Can you work these out from the model? Positions are in its coordinate system, mm. A direction names the side the tool comes from. Round coordinates to 2 decimals unless told otherwise and drop trailing zeros. Loops run counter-clockwise (first coordinate to the right, second up) from the corner with the lowest first, then second, coordinate; pieces in that order, holes last.
```python
from build123d import *

# Parameters (mm, degrees)
SKETCH_W              = 115
SKETCH_H              = 25
PAD_DEPTH             = 3
PAD001_DEPTH          = 3
SKETCH002_W           = 115
SKETCH002_H           = 25
SKETCH002_W_2         = 96
SKETCH002_H_2         = 3
PAD002_DEPTH          = 3
SKETCH003_R           = 0.825
POCKET_DEPTH          = 245.060315
POLARPATTERN_COUNT    = 2
POLARPATTERN001_COUNT = 2
POLARPATTERN002_COUNT = 2
FILLET_R              = 2
SKETCH004_R           = 12.75
POCKET001_DEPTH       = 3
POCKET002_DEPTH       = 3
FILLET001_R           = 0.4
FILLET002_R           = 2


with BuildPart() as part:
    # Sketch → Pad (new body)
    with BuildSketch(Plane.XY):
        Rectangle(SKETCH_W, SKETCH_H)
    extrude(amount=PAD_DEPTH)

    # Sketch001 (on Face6 of Pad) → Pad001 (join)
    with BuildSketch(Plane.XY.offset(3)):
        Polygon((-57.5, 12.5), (57.5, 12.5), (57.5, 4), (50, 4), (50, 5), (-50, 5), (-50, 4), (-57.5, 4), align=None)
        Polygon((-57.5, -12.5), (57.5, -12.5), (57.5, -4), (50, -4), (50, -5), (-50, -5), (-50, -4), (-57.5, -4), align=None)
    extrude(amount=PAD001_DEPTH)

    # Sketch002 (on Face12 of Pad001) → Pad002 (join)
    with BuildSketch(Plane.XY.offset(6)):
        Rectangle(SKETCH002_W, SKETCH002_H)
        Rectangle(SKETCH002_W_2, SKETCH002_H_2, mode=Mode.SUBTRACT)
    extrude(amount=PAD002_DEPTH)

    # Sketch003 (on Face26 of Pad002) → Pocket (cut, through all)
    with BuildSketch(Plane.XY.offset(9)):
        with Locations((-52.5, 7.5)):
            Circle(SKETCH003_R)
    pocket = extrude(amount=-POCKET_DEPTH, mode=Mode.SUBTRACT)

    # PolarPattern: Pocket ×2 about axis
    polarpattern_axis = Axis((0, 0, 0), (0, 1, 0))
    for i in range(1, POLARPATTERN_COUNT):
        add(pocket.rotate(polarpattern_axis, i * 360 / POLARPATTERN_COUNT), mode=Mode.SUBTRACT)

    # PolarPattern001: Pocket ×2 about axis
    polarpattern001_axis = Axis((0, 0, 0), (1, 0, 0))
    for i in range(1, POLARPATTERN001_COUNT):
        add(pocket.rotate(polarpattern001_axis, i * 360 / POLARPATTERN001_COUNT), mode=Mode.SUBTRACT)

    # PolarPattern002: Pocket ×2 about axis
    polarpattern002_axis = Axis((0, 0, 9), (0, 0, 1))
    for i in range(1, POLARPATTERN002_COUNT):
        add(pocket.rotate(polarpattern002_axis, i * 360 / POLARPATTERN002_COUNT), mode=Mode.SUBTRACT)

    # Fillet
    fillet_edges = [part.edges().sort_by_distance(p)[0] for p in [
        (57.5, 12.5, 7.5),
        (57.5, 12.5, 4.5),
        (57.5, 12.5, 1.5),
        (57.5, -12.5, 7.5),
        (-57.5, 12.5, 7.5),
        (-57.5, -12.5, 7.5),
    ]]
    fillet(fillet_edges, radius=FILLET_R)

    # Sketch004 (on Face2 of Fillet) → Pocket001 (cut)
    with BuildSketch(Plane(origin=(0, 0, 0), x_dir=(1, 0, 0), z_dir=(0, 0, -1))):
        with Locations((0, -4.31247)):
            Circle(SKETCH004_R)
    extrude(amount=-POCKET001_DEPTH, mode=Mode.SUBTRACT)

    # Sketch005 (on Face2 of Pocket001) → Pocket002 (cut)
    with BuildSketch(Plane(origin=(0, 0, 0), x_dir=(1, 0, 0), z_dir=(0, 0, -1))):
        Polygon((0.086598, 10.584693), (-49.736099, 10.584693), (-49.736099, 6.30074), (-54.94091, 3.161258), (-54.94091, -2.621142), (-51.300568, -2.835279), (-51.086433, 1.161956), (-44.025761, 5.729707), (0.086598, 5.729707), align=None)
    extrude(amount=-POCKET002_DEPTH, mode=Mode.SUBTRACT)

    # Fillet001
    fillet001_edges = [part.edges().sort_by_distance(p)[0] for p in [
        (-7.856028, -5.729707, 1.5),
    ]]
    fillet(fillet001_edges, radius=FILLET001_R)

    # Fillet002
    fillet002_edges = [part.edges().sort_by_distance(p)[0] for p in [
        (0.086598, -8.437236, 1.5),
    ]]
    fillet(fillet002_edges, radius=FILLET002_R)


solid = part.part
```
(1) Suppose I cut it at A-A (z = 4.25). Write out the boundary of the cut face in (x, y) (3 decimals), then the cut area to 3 significant figures.
(2) For pin 1 (5 mm diameter, centred on x = 2.5, y = 0, fed in from -Z); pin 2 (8.5 mm diameter, centred on x = -4.5, y = 7, fed in from -Z), each with a flat end and sliding along its axis, tell me the tip position at first contact or that it passes through.
(3) Suppose I cut it at B-B (x = -4.5). Write out the boundary of the cut face in (y, z), then the cut area to 3 significant figures.
(4) Which directions (+Z, -Z, +X, -X, +Y, -Y) give clear straight access to the entire face, cutting with the end or side of a thin tool? Please do faces 5 (the flat face through (54, -4, 4)), 6 (the flat face through (-24, -10.585, 1)), 7 (the flat face through (33, 0, 3)).
(5) We'd pull the mould along Z, two halves only. Please class faces 1 (the flat face through (-1, -1.5, 7)), 2 (the flat face through (-1, 3, 9)), 3 (the flat face through (-1, 2, 6)), 4 (the flat face through (1, 5, 4)): released by +Z, released by -Z, zero draft, split by the parting line, or undercut.
(6) If I drill on line 1 (X direction, y = -7.5, z = 5) (3 decimals); line 2 (Y direction, x = 52.5, z = 6.75) (3 decimals); line 3 (Y direction, x = -52.5, z = 4) (3 decimals), over which ranges is the centre line in solid material (lowest first)?
Check result:
1. outline: (-57.5, -10.5) arc R2 ccw to (-55.5, -12.5) - (55.5, -12.5) arc R2 ccw to (57.5, -10.5) - (57.5, -4) - (50, -4) - (50, -5) - (-50, -5) - (-50, -4) - (-57.5, -4) - close; (-57.5, 4) - (-50, 4) - (-50, 5) - (50, 5) - (50, 4) - (57.5, 4) - (57.5, 10.5) arc R2 ccw to (55.5, 12.5) - (-55.5, 12.5) arc R2 ccw to (-57.5, 10.5) - close; hole circle Ø1.65 at (-52.5, -7.5); hole circle Ø1.65 at (-52.5, 7.5); hole circle Ø1.65 at (52.5, -7.5); hole circle Ø1.65 at (52.5, 7.5)
1. area: 1,740 mm2
2. pin 1: stops at z = 6
2. pin 2: stops at z = 3
3. outline: (-12.5, 0) - (-10.58, 0) - (-10.58, 3) - (-5, 3) - (-5, 6) - (-1.5, 6) - (-1.5, 9) - (-12.5, 9) - close; (1.5, 6) - (5, 6) - (5, 3) - (12.5, 3) - (12.5, 9) - (1.5, 9) - close
3. area: 117 mm2
4. face 5: +X, -X
4. face 6: -Z
4. face 7: none
5. face 1: zero draft
5. face 2: released by +Z
5. face 3: undercut
5. face 4: undercut
6. line 1: x = -57.5 to -53.325, -51.675 to 51.675, 53.325 to 57.5
6. line 2: y = -12.5 to -8.325, -6.675 to 6.675, 8.325 to 12.5
6. line 3: y = -12.5 to -8.325, -6.675 to -4, 4 to 6.675, 8.325 to 12.5
